```python
from build123d import *

# Parameters (mm, degrees)
SKETCH1_W                                       = 11
SKETCH1_H                                       = 63
SKETCH1_W_2                                     = 60
SKETCH1_H_2                                     = 60
BOSS_EXTRUDE1_DEPTH                             = 3
CSK_FOR_M3_FLAT_HEAD_MACHINE_SCREW1_D           = 3.6
CSK_FOR_M3_FLAT_HEAD_MACHINE_SCREW1_DEPTH       = 6
CSK_FOR_M3_FLAT_HEAD_MACHINE_SCREW1_CSINK_D     = 6.8
CSK_FOR_M3_FLAT_HEAD_MACHINE_SCREW1_CSINK_ANGLE = 90
CSK_FOR_M3_FLAT_HEAD_MACHINE_SCREW1_TIP         = 1.081549114
FILLET1_R                                       = 5


with BuildPart() as part:
    # Sketch1 → Boss-Extrude1 (new body)
    with BuildSketch(Plane.XY):
        with Locations((-66.5, 31.5)):
            Rectangle(SKETCH1_W, SKETCH1_H)
        Polygon((-60, 60), (0, 60), (0, 63), (-61, 63), (-61, 0), (-60, 0), align=None)
        with Locations((-30, 30)):
            Rectangle(SKETCH1_W_2, SKETCH1_H_2)
        with Locations((5.5, 31.5)):
            Rectangle(SKETCH1_W, SKETCH1_H)
    extrude(amount=BOSS_EXTRUDE1_DEPTH)

    # CSK for M3 Flat Head Machine Screw1
    with Locations(Plane.XY.offset(3)):
        with Locations((-65.5, 31.5), (-65.5, 51.5), (-65.5, 11.5), (4.5, 11.5), (4.5, 31.5), (4.5, 51.5)):
            CounterSinkHole(CSK_FOR_M3_FLAT_HEAD_MACHINE_SCREW1_D / 2, CSK_FOR_M3_FLAT_HEAD_MACHINE_SCREW1_CSINK_D / 2, depth=CSK_FOR_M3_FLAT_HEAD_MACHINE_SCREW1_DEPTH, counter_sink_angle=CSK_FOR_M3_FLAT_HEAD_MACHINE_SCREW1_CSINK_ANGLE)
            with Locations((0, 0, -(CSK_FOR_M3_FLAT_HEAD_MACHINE_SCREW1_DEPTH + CSK_FOR_M3_FLAT_HEAD_MACHINE_SCREW1_TIP / 2))):  # 118° drill point
                Cone(0, CSK_FOR_M3_FLAT_HEAD_MACHINE_SCREW1_D / 2, CSK_FOR_M3_FLAT_HEAD_MACHINE_SCREW1_TIP, mode=Mode.SUBTRACT)

    # Fillet1
    fillet1_edges = [part.edges().sort_by_distance(p)[0] for p in [
        (11, 0, 1.5),
        (-72, 0, 1.5),
    ]]
    fillet(fillet1_edges, radius=FILLET1_R)


solid = part.part
```
Can you work these out from the model? Positions are in its coordinate system, mm. Give positions to 0.01 mm unless a question says otherwise; leave off trailing zeros. Loops run counter-clockwise (first coordinate to the right, second up) from the corner with the lowest first, then second, coordinate; pieces in that order, holes last. Notation, with made-up numbers: M 29.5,56 L 88.5,56 A33 cw 88.5,91 Z; hole C 84,-24.75 d5. An arc over 180 degrees is marked long. Answer in a Markdown table with one row per item.
1. Suppose I cut it at A-A on x = -65.5. Write out the boundary of the cut face in (y, z), plus the area to 3 significant figures.
Taken from the geometry:
| item | result |
|---|---|
| outline | M 0,0 L 9.7,0 L 9.7,1.4 L 8.1,3 L 0,3 Z; M 13.3,0 L 29.7,0 L 29.7,1.4 L 28.1,3 L 14.9,3 L 13.3,1.4 Z; M 33.3,0 L 49.7,0 L 49.7,1.4 L 48.1,3 L 34.9,3 L 33.3,1.4 Z; M 53.3,0 L 63,0 L 63,3 L 54.9,3 L 53.3,1.4 Z |
| area | 149 mm² |
2. For pin 1 Ø2 at (x, y) = (4.5, 11.5) entering from -Z; pin 2 Ø4.5 at (x, y) = (4.5, 31.5) entering from -Z, each with a flat end and sliding along its axis, tell me the tip position at first contact or that it passes through.
Taken from the geometry:
| item | result |
|---|---|
| pin 1 | passes through |
| pin 2 | stops at z = 0 |
3. If I drill on line 1 along Y through (x, z) = (-65.5, 0.3); line 2 along X through (y, z) = (31.5, 0.4); line 3 along Y through (x, z) = (-63.5, 2.15), over which ranges is the centre line in solid material (lowest first)?
Taken from the geometry:
| item | result |
|---|---|
| line 1 | y = 0 to 9.7, 13.3 to 29.7, 33.3 to 49.7, 53.3 to 63 |
| line 2 | x = -72 to -67.3, -63.7 to 2.7, 6.3 to 11 |
| line 3 | y = 0 to 9.92, 13.08 to 29.92, 33.08 to 49.92, 53.08 to 63 |
4. Suppose I cut it at C-C on z = 2.3. Write out the boundary of the cut face in (x, y).
Taken from the geometry:
| item | result |
|---|---|
| outline | M -72,5 A5 ccw -67,0 L 6,0 A5 ccw 11,5 L 11,63 L -72,63 Z; hole C -65.5,11.5 d5.4; hole C -65.5,31.5 d5.4; hole C -65.5,51.5 d5.4; hole C 4.5,11.5 d5.4; hole C 4.5,31.5 d5.4; hole C 4.5,51.5 d5.4 |
5. Thinking about a two-plate mould opening in X: for faces 1 (the flat face through (11, 34, 1)), 2 (the flat face through (-31, 32, 0)), 3 (the cylindrical face through (2.783, 12.041, 0.69)), which applies, released by +X, released by -X, zero draft, split by the parting line, or undercut?
Taken from the geometry:
| item | result |
|---|---|
| face 1 | released by +X |
| face 2 | zero draft |
| face 3 | undercut |
6. Suppose I cut it at B-B on y = 31.5. Write out the boundary of the cut face in (x, z).
Taken from the geometry:
| item | result |
|---|---|
| outline | M -72,0 L -67.3,0 L -67.3,1.4 L -68.9,3 L -72,3 Z; M -63.7,0 L 2.7,0 L 2.7,1.4 L 1.1,3 L -62.1,3 L -63.7,1.4 Z; M 6.3,0 L 11,0 L 11,3 L 7.9,3 L 6.3,1.4 Z |
